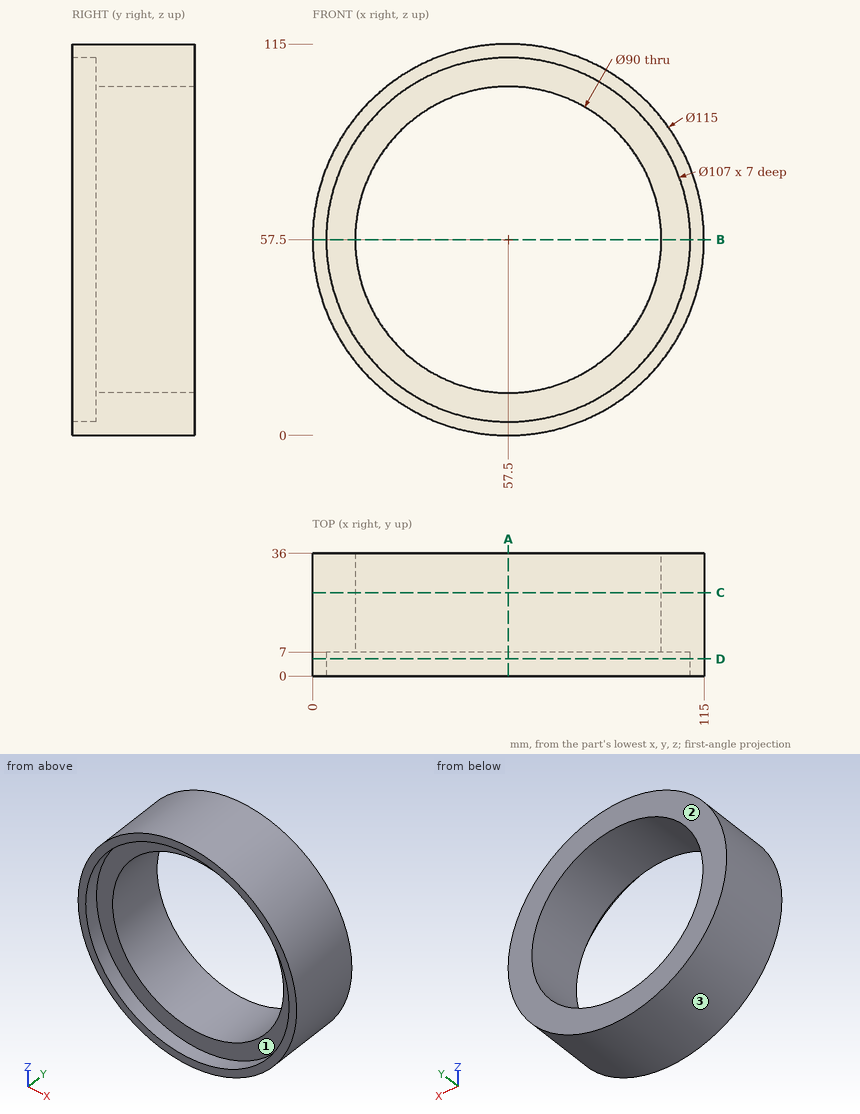
Design review of the part shown in the three views and the two pictorial views. Dimensions are in mm from the part's minimum x, y and z. Round coordinates to 2 decimals unless told otherwise and drop trailing zeros. Order: outer loops, then holes, each group sorted by start corner. A loop starts at its lowest first (then second) coordinate and runs counter-clockwise, first axis right, second up. Notation, with made-up numbers: M -30,8 L 8,8 A24 cw 8,30 Z; hole C 45,-20 d8. An arc over 180 degrees is marked long. Put each result on its own line as item: value.
Q1. Consider section C-C (y = 24.5). State the section outline as (x, z) points, and give its area (3 significant figures).
Reported:
outline: C 57.5,57.5 d115; hole C 57.5,57.5 d90
area: 4,030 mm²
Q2. To check wall thickness, follow line 1 (Z direction, x = 57, y = 18); line 2 (Y direction, x = 34, z = 15); line 3 (X direction, y = 15, z = 60). State the ranges of each line that lie inside material, in increasing order.
Reported:
line 1: 0 to 12.5, 102.5 to 115
line 2: 7 to 36
line 3: 0.05 to 12.57, 102.43 to 114.95
Q3. Consider section D-D (y = 5). State the section outline as (x, z) points.
Reported:
outline: C 57.5,57.5 d115; hole C 57.5,57.5 d107
Q4. Consider section A-A (x = 57.5). State the section outline as (y, z) points.
Reported:
outline: M 0,0 L 36,0 L 36,12.5 L 7,12.5 L 7,4 L 0,4 Z; M 0,111 L 7,111 L 7,102.5 L 36,102.5 L 36,115 L 0,115 Z
Q5. Draft analysis for pull direction Z (two halves, no side actions). For the marked faces 1, 2 and 3, state which applies: released by +Z, released by -Z, zero draft, split by the parting line, or undercut.
Reported:
face 1: undercut
face 2: zero draft
face 3: split by the parting line
Q6. Insertion check: pin 1 Ø3 at (y, z) = (9, 20.5) entering from -X; pin 2 Ø1 at (x, y) = (14, 18) entering from +Z; pin 3 Ø4 at (y, z) = (5, 99.5) entering from +X. Each pin has a flat end and moves straight along its axis. Give the tip position at first contact, or say it passes through.
Reported:
pin 1: x = 12.27
pin 2: z = 95.67
pin 3: x = 98.81
Q7. Consider section B-B (z = 57.5). State the section outline as (x, y) points.
Reported:
outline: M 0,0 L 4,0 L 4,7 L 12.5,7 L 12.5,36 L 0,36 Z; M 102.5,7 L 111,7 L 111,0 L 115,0 L 115,36 L 102.5,36 Z
